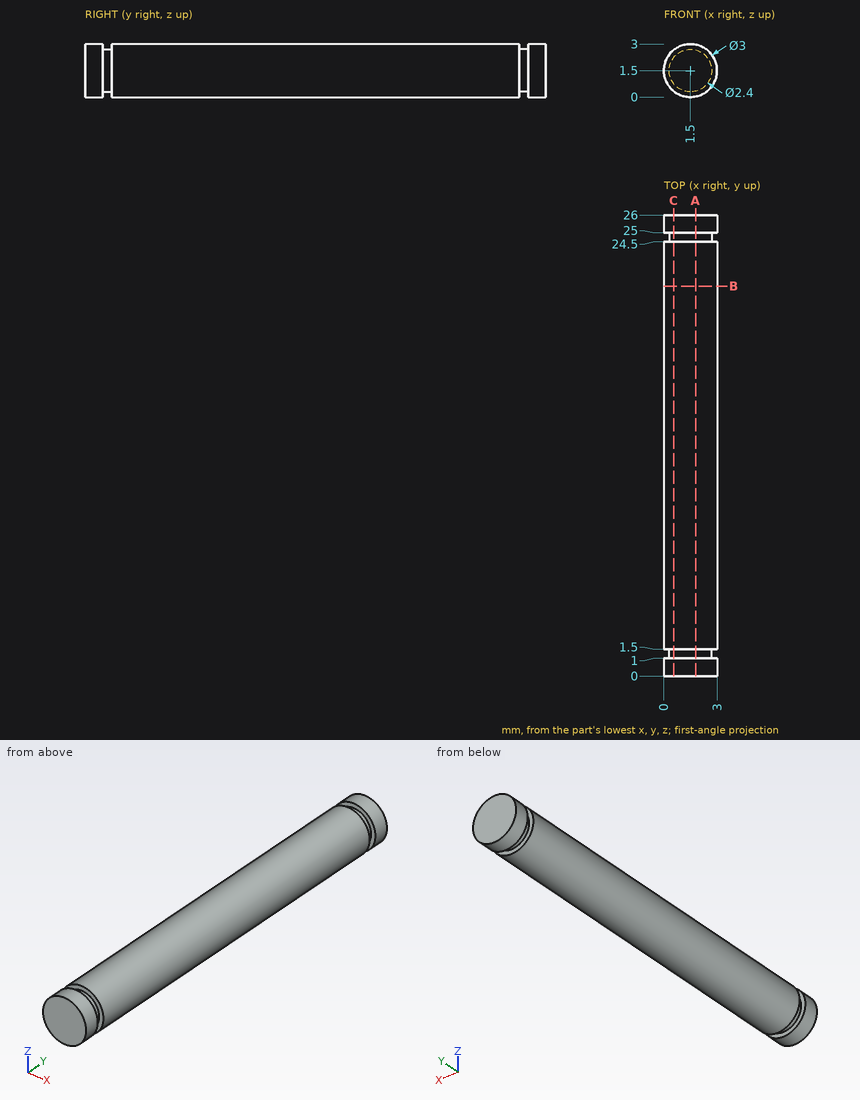
Part print with two shaded views. Sizes in mm from the minimum x, y, z corner. Round coordinates to 2 decimals unless told otherwise and drop trailing zeros. Write each loop counter-clockwise with the first axis right and the second up, starting at its lowest first coordinate (ties: lowest second). Pieces come first, ordered by that corner, then holes. Notation, with made-up numbers: M 63.25,-35 L 80.25,-35 A22 ccw 80.25,-27 Z; hole C -6.75,-13.75 d8. An arc over 180 degrees is marked long. Put each result on its own line as item: value. Start each with the question number.
1) Pin check, flat tip, straight feed: pin 1 Ø1.5 at (x, y) = (0.5, 12) entering from +Z. Stop position of the tip, or through.
2) Saw through at A-A, the plane x = 1.8. Write the cut outline in (y, z).
3) Saw through at B-B, the plane y = 22. Write the cut outline in (x, z).
4) Drill centre lines: probe 1 along Y at (x, z) = (2.15, 2.55); probe 2 along Z at (x, y) = (1.6, 13.5); probe 3 along X at (y, z) = (23.75, 1.9). Where is each one in solid material? Low to high. Write a range as [from, to].
5) Saw through at C-C, the plane x = 0.55. Write the cut outline in (y, z).
Resolved:
1. pin 1: z = 2.98
2. outline: M 0,0.03 L 1,0.03 L 1,0.34 L 1.5,0.34 L 1.5,0.03 L 24.5,0.03 L 24.5,0.34 L 25,0.34 L 25,0.03 L 26,0.03 L 26,2.97 L 25,2.97 L 25,2.66 L 24.5,2.66 L 24.5,2.97 L 1.5,2.97 L 1.5,2.66 L 1,2.66 L 1,2.97 L 0,2.97 Z
3. outline: C 1.5,1.5 d3
4. probe 1: [0, 1], [1.5, 24.5], [25, 26]
4. probe 2: [0, 3]
4. probe 3: [0.05, 2.95]
5. outline: M 0,0.34 L 1,0.34 L 1,0.77 L 1.5,0.77 L 1.5,0.34 L 24.5,0.34 L 24.5,0.77 L 25,0.77 L 25,0.34 L 26,0.34 L 26,2.66 L 25,2.66 L 25,2.23 L 24.5,2.23 L 24.5,2.66 L 1.5,2.66 L 1.5,2.23 L 1,2.23 L 1,2.66 L 0,2.66 Z
